```python
from build123d import *

# Parameters (mm, degrees)
SKETCH2_W           = 15
SKETCH2_H           = 30.5
SKETCH2_W_2         = 7.5
SKETCH2_H_2         = 30
SKETCH2_W_3         = 45
SKETCH2_W_4         = 30
SKETCH2_H_3         = 12
BOSS_EXTRUDE1_DEPTH = 3
SKETCH3_W           = 15
SKETCH3_H           = 6
BOSS_EXTRUDE2_DEPTH = 23
SKETCH4_R           = 1.6
CUT_EXTRUDE1_DEPTH  = 23
SKETCH5_R           = 4.6
CUT_EXTRUDE2_DEPTH  = 23
SKETCH6_R           = 1.6
CUT_EXTRUDE3_DEPTH  = 23
CHAMFER1_SIZE       = 1
FILLET1_R           = 1
CHAMFER2_SIZE       = 5


with BuildPart() as part:
    # Sketch2 → Boss-Extrude1 (new body)
    with BuildSketch(Plane(origin=(0, 0, 0), x_dir=(1, 0, 0), z_dir=(0, 1, 0))):
        with Locations((-67.5, -42.25)):
            Rectangle(SKETCH2_W, SKETCH2_H)
        Polygon((-60, 57.5), (-75, 57.5), (-75, -27), (-60, -27), (-60, -15), (-67.5, -15), (-67.5, 15), (-60, 15), (-60, 27), align=None)
        with Locations((-63.75, 0)):
            Rectangle(SKETCH2_W_2, SKETCH2_H_2)
        with Locations((-37.5, 0)):
            Rectangle(SKETCH2_W_3, SKETCH2_H_2)
        Rectangle(SKETCH2_W_4, SKETCH2_H_2)
        Polygon((-15, 27), (-15, 15), (15, 15), (15, 27), (-17.5, 43.5), (-27.5, 43.5), align=None)
        Polygon((-27.5, -43.5), (-15, -27), (15, -27), (-17.5, -43.5), align=None)
        with Locations((0, -21)):
            Rectangle(SKETCH2_W_4, SKETCH2_H_3)
        with Locations((37.5, 0)):
            Rectangle(SKETCH2_W_3, SKETCH2_H_2)
        with Locations((63.75, 0)):
            Rectangle(SKETCH2_W_2, SKETCH2_H_2)
        Polygon((60, 27), (60, 15), (67.5, 15), (67.5, -15), (60, -15), (60, -27), (75, -27), (75, 57.5), (60, 57.5), align=None)
        with Locations((67.5, -42.25)):
            Rectangle(SKETCH2_W, SKETCH2_H)
    extrude(amount=BOSS_EXTRUDE1_DEPTH)

    # Sketch3 → Boss-Extrude2 (add)
    with BuildSketch(Plane(origin=(0, 3, 0), x_dir=(1, 0, 0), z_dir=(0, 1, 0))):
        with Locations((-67.5, 54.5)):
            Rectangle(SKETCH3_W, SKETCH3_H)
        Polygon((-17.5, 43.5), (-27.5, 43.5), (-25.984848485, 41.5), (-13.560606061, 41.5), align=None)
        with Locations((67.5, 54.5)):
            Rectangle(SKETCH3_W, SKETCH3_H)
    extrude(amount=BOSS_EXTRUDE2_DEPTH)

    # Sketch4 → Cut-Extrude1 (cut)
    with BuildSketch(Plane(origin=(0, 0, -43.5), x_dir=(-1, 0, 0), z_dir=(0, 0, -1))):
        with Locations((22.5, 23.25)):
            Circle(SKETCH4_R)
        with Locations((22.5, 5.75)):
            Circle(SKETCH4_R)
    extrude(amount=-CUT_EXTRUDE1_DEPTH, mode=Mode.SUBTRACT)

    # Sketch5 → Cut-Extrude2 (cut)
    with BuildSketch(Plane(origin=(0, 0, -57.5), x_dir=(-1, 0, 0), z_dir=(0, 0, -1))):
        with Locations((67.5, 14.5)):
            Circle(SKETCH5_R)
    cut_extrude2 = extrude(amount=-CUT_EXTRUDE2_DEPTH, mode=Mode.SUBTRACT)

    # Mirror3: Cut-Extrude2 across plane
    add(cut_extrude2.mirror(Plane(origin=(0, 0, 0), x_dir=(0, 0, 1), z_dir=(1, 0, 0))), mode=Mode.SUBTRACT)

    # Mirror4: part across plane


with BuildPart() as part_1:
    add(part.part)
    add(part.part.mirror(Plane.XY))

    # Sketch6 → Cut-Extrude3 (cut)
    with BuildSketch(Plane(origin=(0, 3, 0), x_dir=(1, 0, 0), z_dir=(0, 1, 0))):
        with Locations((-67.5, 27.6)):
            Circle(SKETCH6_R)
        with Locations((0, 27.6)):
            Circle(SKETCH6_R)
        with Locations((67.5, 27.6)):
            Circle(SKETCH6_R)
        with Locations((67.5, -27.6)):
            Circle(SKETCH6_R)
        with Locations((0, -27.6)):
            Circle(SKETCH6_R)
        with Locations((-67.5, -27.6)):
            Circle(SKETCH6_R)
    extrude(amount=-CUT_EXTRUDE3_DEPTH, mode=Mode.SUBTRACT)

    # Chamfer1
    chamfer1_edges = [part_1.edges().sort_by_distance(p)[0] for p in [
        (-67.5, 0, 57.5),
        (-75, 0, 0),
        (-67.5, 0, -57.5),
        (-60, 0, -36.25),
        (-37.5, 0, -15),
        (-15, 0, -21),
        (-21.25, 0, -35.25),
        (-22.5, 0, -43.5),
        (-1.25, 0, -35.25),
        (15, 0, -21),
        (37.5, 0, -15),
        (60, 0, -36.25),
        (67.5, 0, -57.5),
        (75, 0, 0),
        (67.5, 0, 57.5),
        (60, 0, 36.25),
        (37.5, 0, 15),
        (15, 0, 21),
        (-1.25, 0, 35.25),
        (-22.5, 0, 43.5),
        (-21.25, 0, 35.25),
        (-15, 0, 21),
        (-37.5, 0, 15),
        (-60, 0, 36.25),
    ]]
    chamfer(chamfer1_edges, length=CHAMFER1_SIZE)

    # Fillet1
    fillet1_edges = [part_1.edges().sort_by_distance(p)[0] for p in [
        (60, 26, 54.5),
        (75, 26, 54.5),
        (67.5, 26, 51.5),
        (67.5, 26, 57.5),
        (75, 26, -54.5),
        (60, 26, -54.5),
        (67.5, 26, -51.5),
        (67.5, 26, -57.5),
        (-67.5, 26, -57.5),
        (-60, 26, -54.5),
        (-67.5, 26, -51.5),
        (-75, 26, -54.5),
        (-75, 26, 54.5),
        (-60, 26, 54.5),
        (-67.5, 26, 51.5),
        (-67.5, 26, 57.5),
    ]]
    fillet(fillet1_edges, radius=FILLET1_R)

    # Chamfer2
    chamfer2_edges = [part_1.edges().sort_by_distance(p)[0] for p in [
        (-67.5, 3, 51.5),
        (67.5, 3, 51.5),
        (67.5, 3, -51.5),
        (-67.5, 3, -51.5),
    ]]
    chamfer(chamfer2_edges, length=CHAMFER2_SIZE)


solid = part_1.part
```
CAD build for the part. Positions are in the model's coordinates, mm. A direction names the side the tool comes from. Round coordinates to 2 decimals unless told otherwise and drop trailing zeros. Write each loop counter-clockwise with the first axis right and the second up, starting at its lowest first coordinate (ties: lowest second). Pieces come first, ordered by that corner, then holes. Notation, with made-up numbers: (27, 8.25) -> (53, 8.25) arc R17 ccw to (53, 14.25) -> close; hole circle Ø10 at (46, 55). An arc over 180 degrees is marked (long way). Answer in a Markdown table with one row per item. Add a question column.
Item 1: Saw through at D-D, the plane z = -8.5. Write the cut outline in (x, y).
Item 2: Drill centre lines: line 1 (Y direction, x = -22.5, z = -42.1); line 2 (X direction, y = 0.9, z = -27.6); line 3 (Z direction, x = -19.5, y = 16). Where is each one in solid material? Low to high. Write a range as from..to.
Item 3: Which spindle directions (+Z, -Z, +X, -X, +Y, -Y) get a long thin tool onto all of the face, cutting with end or side? Do faces 5 (the face through (75, 2, 0)), 6 (the face through (67, 20, -51.5)), 7 (the face through (60, 9, -52)), 8 (the face through (-0.35, 1.52, 29.16)), 9 (the face through (-60, 9, 52)). Say none if no direction does.
Item 4: Mould opens along Z. For faces 1 (the face through (-1.246, 0.507, 34.695)), 2 (the face through (-62.904, 14.702, 54.542)), 3 (the face through (-67.6, 5.5, 49)), 4 (the face through (-71, 10, -57.5)) say: pulls with the +Z half, pulls with the -Z half, needs draft (parallel to the pull), parting line crosses it, or undercut.
Item 5: Saw through at A-A, the plane x = -67.5. Count the separate pieces of the cut face and the enclosed holes in it, then the cut area to 3 significant figures.
Item 6: Drop flat-ended pins along their axis: pin 1 Ø1 at (x, y) = (-46.5, 1.5) entering from -Z; pin 2 Ø3.5 at (x, z) = (67.5, -27.6) entering from +Y; pin 3 Ø2.5 at (x, z) = (0, -27.6) entering from -Y; pin 4 Ø7 at (y, z) = (15.5, 43.5) entering from -X. Give the stop position or say it passes through.
Item 7: Saw through at C-C, the plane z = -34.5. Write the cut outline in (x, y).
Findings below:
| question | item | result |
|---|---|---|
| 1 | outline | (-75, 1) -> (-74, 0) -> (74, 0) -> (75, 1) -> (75, 3) -> (-75, 3) -> close |
| 2 | line 1 | y = 0..4.15, 7.35..21.65, 24.85..26 |
| 2 | line 2 | x = -74.9..-69.1, -65.9..-60.1, -15.33..-1.6, 1.6..13.6, 60.1..65.9, 69.1..74.9 |
| 2 | line 3 | z = -43.5..-41.5, 41.5..43.5 |
| 3 | face 5 | +Z, -Z, +X, +Y, -Y |
| 3 | face 6 | +X, -X, +Y |
| 3 | face 7 | -Z, +Y, -Y |
| 3 | face 8 | +Y, -Y |
| 3 | face 9 | +Z, +Y, -Y |
| 4 | face 1 | pulls with the +Z half |
| 4 | face 2 | needs draft |
| 4 | face 3 | undercut |
| 4 | face 4 | pulls with the -Z half |
| 5 | separate pieces | 5 |
| 5 | enclosed holes | 0 |
| 5 | area | 515 mm^2 |
| 6 | pin 1 | stops at z = -15 |
| 6 | pin 2 | stops at y = 3 |
| 6 | pin 3 | passes through |
| 6 | pin 4 | stops at x = -27.5 |
| 7 | outline | (-75, 1) -> (-74, 0) -> (-61, 0) -> (-60, 1) -> (-60, 3) -> (-75, 3) -> close; (-20.68, 1) -> (-19.43, 0) -> (-1.98, 0) -> (0.23, 1) -> (0.23, 3) -> (-20.68, 3) -> close; (60, 1) -> (61, 0) -> (74, 0) -> (75, 1) -> (75, 3) -> (60, 3) -> close |
